Geometry check sheet. Reference: drawing and pictorial views, mm from the part's lowest x, y, z. Give positions to 0.01 mm unless a question says otherwise; leave off trailing zeros. Write each loop counter-clockwise with the first axis right and the second up, starting at its lowest first coordinate (ties: lowest second). Pieces come first, ordered by that corner, then holes. Notation, with made-up numbers: M 59,-23.75 L 71,-23.75 A13 ccw 71,-3.75 Z; hole C -1,66.5 d6. An arc over 180 degrees is marked long. Write item = value, one per line. Start each with the question number.
1) Cross-section at D-D, the plane z = 12. Record the cut outline in (x, y).
2) Cross-section at B-B, the plane x = 20. Record the cut outline in (y, z), plus the area to 3 significant figures.
3) Cross-section at C-C, the plane y = 0.7. Record the cut outline in (x, z), plus the area to 3 significant figures.
4) Cross-section at A-A, the plane z = 32.5. Record the cut outline in (x, y).
5) Go/stop test with a flat-tipped pin: pin 1 (1 mm diameter, centred on x = 30.5, z = 13, fed in from +Y). Record where the tip stops, or that it passes through.
6) Scan lines: line 1 along X through (y, z) = (0.4, 39.5); line 2 along X through (y, z) = (0.5, 12); line 3 along Z through (x, y) = (32.5, 0.7). Record each from-to range of solid material in increasing order. Write a range as [from, to].
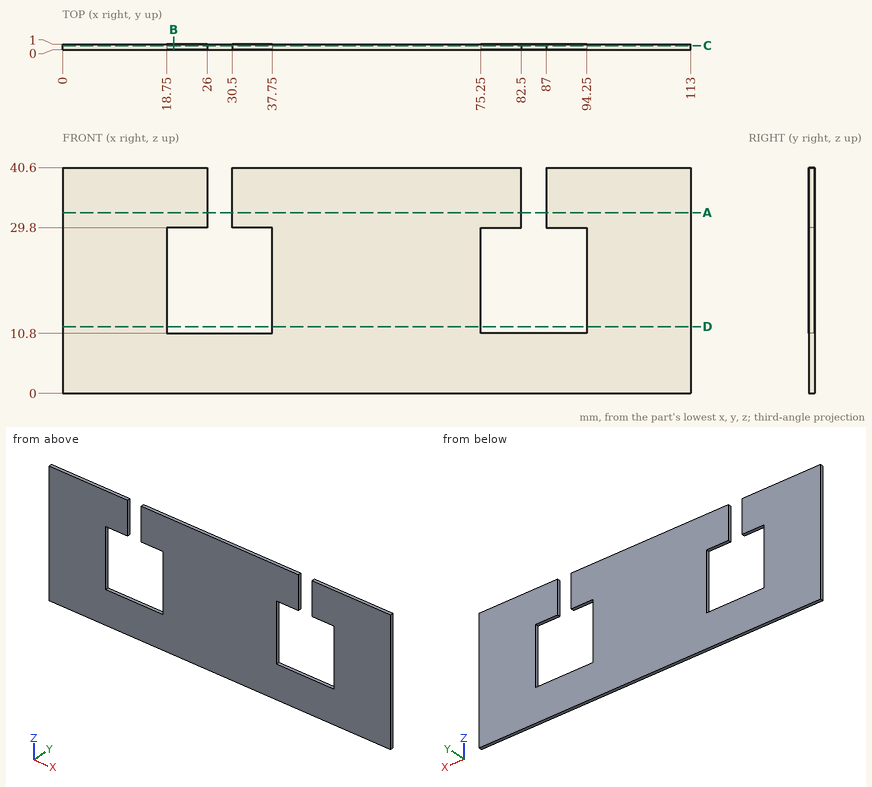
Reply:
q1.outline = M 0,0 L 18.75,0 L 18.75,1 L 0,1 Z; M 37.75,0 L 75.25,0 L 75.25,1 L 37.75,1 Z; M 94.25,0 L 113,0 L 113,1 L 94.25,1 Z
q2.outline = M 0,0 L 1,0 L 1,10.8 L 0,10.8 Z; M 0,29.8 L 1,29.8 L 1,40.6 L 0,40.6 Z
q2.area = 21.6 mm2
q3.outline = M 0,0 L 113,0 L 113,40.6 L 87,40.6 L 87,29.8 L 94.25,29.8 L 94.25,10.8 L 75.25,10.8 L 75.25,29.8 L 82.5,29.8 L 82.5,40.6 L 30.5,40.6 L 30.5,29.8 L 37.75,29.8 L 37.75,10.8 L 18.75,10.8 L 18.75,29.8 L 26,29.8 L 26,40.6 L 0,40.6 Z
q3.area = 3,770 mm2
q4.outline = M 0,0 L 26,0 L 26,1 L 0,1 Z; M 30.5,0 L 82.5,0 L 82.5,1 L 30.5,1 Z; M 87,0 L 113,0 L 113,1 L 87,1 Z
q5.pin_1 = through
q6.line_1 = [0, 26], [30.5, 82.5], [87, 113]
q6.line_2 = [0, 18.75], [37.75, 75.25], [94.25, 113]
q6.line_3 = [0, 10.8], [29.8, 40.6]
